Part model, mm, in its own coordinate system. A direction names the side the tool comes from. Give positions to 0.01 mm unless a question says otherwise; leave off trailing zeros. Write each loop counter-clockwise with the first axis right and the second up, starting at its lowest first coordinate (ties: lowest second). Pieces come first, ordered by that corner, then holes. Notation, with made-up numbers: M -11,-17 L 17,-17 A21 ccw 17,8 Z; hole C 38.5,75 d6. An arc over 180 degrees is marked long. Answer as CSV lines item,"result". Start each with the question number.
1) Wall check: line 1 along Z through (x, y) = (-1.55, 0.7); line 2 along Y through (x, z) = (1.25, -2.25); line 3 along X through (y, z) = (-1.15, -1). Give the ranges that are in metal, low to high. Write a range as from..to.
2) Slice it at B-B, the plane z = -10.75. Give the cut face in (x, y), plus the area to 3 significant figures.
3) Slice it at A-A, the plane x = 0. Give the cut face in (y, z).
4) Tool access for faces 4 (the flat face through (0, -2, -3)), 5 (the cylindrical face through (-0.596, -2.685, -1.582)), 6 (the flat face through (1.088, 0.616, -0.542)): list every direction of +Z, -Z, +X, -X, +Y, -Y with a clear straight run to the whole face (end or side of a thin tool).
5) Slice it at C-C, the plane z = -2.75. Give the cut face in (x, y), plus the area to 3 significant figures.
6) Pin check, flat tip, straight feed: pin 1 Ø3 at (y, z) = (1, -5) entering from +X. Stop position of the tip, or through.
7) Mould opens along X. For faces 1 (the flat face through (0.79, 0.44, -1.3)), 2 (the flat face through (1.1, -1.1, 0)), 3 (the cylindrical face through (-1.5, 0.07, -7.78)) say: pulls with the +X half, pulls with the -X half, needs draft (parallel to the pull), parting line crosses it, or undercut.
```python
from build123d import *

# Parameters (mm, degrees)
F3_DEPTH = 1.6
F4_SIZE2 = 0.8660254038
F4_SIZE  = 0.5
F5_SIZE  = 0.3
F6_R     = 0.1


with BuildPart() as f1:
    # F0 (on Front) → F1 (revolve)
    with BuildSketch(Plane.XZ):
        Polygon((2.75, 0), (0, 0), (0, -13), (1.5, -13), (1.5, -3), (2.75, -3), align=None)
    revolve(axis=Axis((0, 0, -6.5), (0, 0, 1)))

    # F2 (on face) → F3 (cut)
    with BuildSketch(Plane.XY):
        Polygon((0.7216878365, 1.25), (-0.7216878365, 1.25), (-1.443375673, 0), (-0.7216878365, -1.25), (0.7216878365, -1.25), (1.443375673, 0), align=None)
    extrude(amount=-F3_DEPTH, mode=Mode.SUBTRACT)

    # F4
    f4_edges = [f1.edges().sort_by_distance(p)[0] for p in [
        (0, 1.25, -1.6),
        (-1.082532, 0.625, -1.6),
        (-1.082532, -0.625, -1.6),
        (0, -1.25, -1.6),
        (1.082532, -0.625, -1.6),
        (1.082532, 0.625, -1.6),
    ]]
    chamfer(f4_edges, length=F4_SIZE, length2=F4_SIZE2)

    # F5
    f5_edges = [f1.edges().sort_by_distance(p)[0] for p in [
        (-2.75, 0, 0),
        (-1.5, 0, -13),
    ]]
    chamfer(f5_edges, length=F5_SIZE)

    # F6
    f6_edges = [f1.edges().sort_by_distance(p)[0] for p in [
        (-2.75, 0, -3),
    ]]
    fillet(f6_edges, radius=F6_R)


with BuildPart() as f7_1:
    # F7: copy of F1
    add(f1.part)


solid = f1.part
```
Found:
1,line 1,"-3..0"
1,line 2,"-2.45..2.45"
1,line 3,"-2.5..-0.78, 0.78..2.5"
2,outline,"C 0,0 d3"
2,area,"7.07 mm²"
3,outline,"M -2.75,-2.9 A0.1 ccw -2.65,-3 L -1.5,-3 L -1.5,-12.7 L -1.2,-13 L 1.2,-13 L 1.5,-12.7 L 1.5,-3 L 2.65,-3 A0.1 ccw 2.75,-2.9 L 2.75,-0.3 L 2.45,0 L 1.25,0 L 1.25,-1.1 L 0.38,-1.6 L -0.38,-1.6 L -1.25,-1.1 L -1.25,0 L -2.45,0 L -2.75,-0.3 Z"
4,face 4,"-Z"
4,face 5,"+Z, -Z"
4,face 6,"+Z"
5,outline,"C 0,0 d5.5"
5,area,"23.8 mm²"
6,pin 1,"x = 1.5"
7,face 1,"undercut"
7,face 2,"needs draft"
7,face 3,"parting line crosses it"
